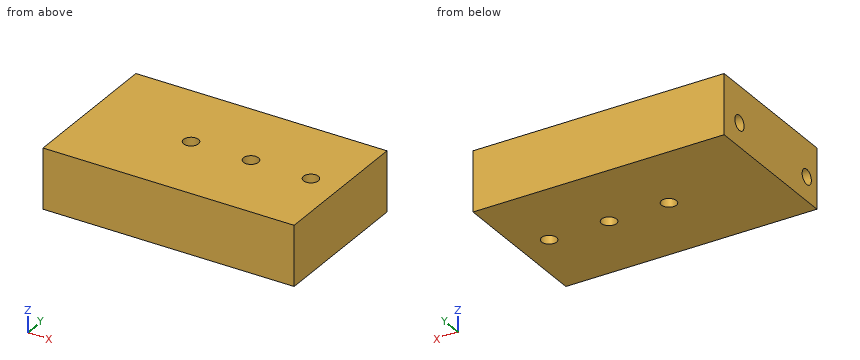
```python
from build123d import *

# Parameters (mm, degrees)
SKETCH1_W                   = 25.4
SKETCH1_H                   = 63.5
BOSS_EXTRUDE1_DEPTH         = 106.37596
F_1_4_0_25_DIAMETER_HOLE1_D = 6.35
F_6_0MM_DOWEL_HOLE1_D       = 6.3
F_6_0MM_DOWEL_HOLE1_DEPTH   = 9.0000074
F_6_0MM_DOWEL_HOLE1_TIP     = 1.89271095


with BuildPart() as part:
    # Sketch1 → Boss-Extrude1 (new body)
    with BuildSketch(Plane(origin=(0, 0, 0), x_dir=(0, 0, -1), z_dir=(1, 0, 0))):
        with Locations((12.7, 31.75)):
            Rectangle(SKETCH1_W, SKETCH1_H)
    extrude(amount=BOSS_EXTRUDE1_DEPTH)

    # 1/4 (0.25) Diameter Hole1 (through all)
    with Locations(Plane.XY):
        with Locations((42.87596001, 32), (93.67596001, 32), (68.27596001, 32)):
            Hole(F_1_4_0_25_DIAMETER_HOLE1_D / 2)

    # Ø6.0mm Dowel Hole1
    with Locations(Plane.ZY):
        with Locations((-15.4, 7), (-15.4, 53)):
            Hole(F_6_0MM_DOWEL_HOLE1_D / 2, depth=F_6_0MM_DOWEL_HOLE1_DEPTH)
            with Locations((0, 0, -(F_6_0MM_DOWEL_HOLE1_DEPTH + F_6_0MM_DOWEL_HOLE1_TIP / 2))):  # 118° drill point
                Cone(0, F_6_0MM_DOWEL_HOLE1_D / 2, F_6_0MM_DOWEL_HOLE1_TIP, mode=Mode.SUBTRACT)


solid = part.part
```
Work out the finished part from the listing and answer in its coordinate system (mm). Round coordinates to 2 decimals unless told otherwise and drop trailing zeros. Write each loop counter-clockwise with the first axis right and the second up, starting at its lowest first coordinate (ties: lowest second). Pieces come first, ordered by that corner, then holes. Notation, with made-up numbers: (38.5, 60.25) -> (86.5, 60.25) arc R22 ccw to (86.5, 96.25) -> close; hole circle Ø9 at (-34.75, -16). An arc over 180 degrees is marked (long way). Write each question's results on one line, items separated by ' | '.
Q1. A flat-ended cylindrical pin translates along its axis: P1, Ø5.5, axis at x = 42.88, y = 32, coming from the +Z side. Find the tip coordinate at first contact, or state that the pin passes through.
Data:
P1: through
Q2. Section A-A, the plane y = 32 is taken. Write down the section's boundary in (x, z), then the cut area to 3 significant figures.
Data:
outline: (0, -25.4) -> (39.7, -25.4) -> (39.7, 0) -> (0, 0) -> close; (46.05, -25.4) -> (65.1, -25.4) -> (65.1, 0) -> (46.05, 0) -> close; (71.45, -25.4) -> (90.5, -25.4) -> (90.5, 0) -> (71.45, 0) -> close; (96.85, -25.4) -> (106.38, -25.4) -> (106.38, 0) -> (96.85, 0) -> close | area: 2,220 mm^2
Q3. Straight lines are drawn through the part: line 1 along Y through (x, z) = (5.75, -15.4); line 2 along Z through (x, y) = (3, 7); line 3 along Y through (x, z) = (4, -13.75). For each, find the intervals that lie inside material, in ascending order. Write a range as [from, to].
Data:
line 1: [0, 3.85], [10.15, 49.85], [56.15, 63.5] | line 2: [-25.4, -18.55], [-12.25, 0] | line 3: [0, 4.32], [9.68, 50.32], [55.68, 63.5]
Q4. Section B-B, the plane z = -17 is taken. Give the number of separate pieces and of enclosed holes in the cut face, then the cut area to 3 significant figures.
Data:
separate pieces: 1 | enclosed holes: 3 | area: 6,560 mm^2
